from build123d import *

# Parameters (mm, degrees)
SKETCH1_W           = 15.5
SKETCH1_H           = 15.5
BOSS_EXTRUDE1_DEPTH = 6.4
FILLET1_R           = 2.54
FILLET2_R           = 2.54
FILLET3_R           = 2.54
FILLET4_R           = 2.54
SKETCH2_W           = 11
SKETCH2_H           = 11
BOSS_EXTRUDE2_DEPTH = 4
SKETCH3_R           = 5.1
BOSS_EXTRUDE3_DEPTH = 22.9
SKETCH4_W           = 0.7
SKETCH4_H           = 2.8
BOSS_EXTRUDE4_DEPTH = 5.8
CUT_EXTRUDE1_DEPTH  = 35.312716302


with BuildPart() as part:
    # Sketch1 → Boss-Extrude1 (new body)
    with BuildSketch(Plane(origin=(0, 0, 0), x_dir=(1, 0, 0), z_dir=(0, 1, 0))):
        with Locations((7.75, 7.75)):
            Rectangle(SKETCH1_W, SKETCH1_H)
    extrude(amount=BOSS_EXTRUDE1_DEPTH)

    # Fillet1
    fillet1_edges = [part.edges().sort_by_distance(p)[0] for p in [
        (15.5, 3.2, 0),
    ]]
    fillet(fillet1_edges, radius=FILLET1_R)

    # Fillet2
    fillet2_edges = [part.edges().sort_by_distance(p)[0] for p in [
        (0, 3.2, 0),
    ]]
    fillet(fillet2_edges, radius=FILLET2_R)

    # Fillet3
    fillet3_edges = [part.edges().sort_by_distance(p)[0] for p in [
        (15.5, 3.2, -15.5),
    ]]
    fillet(fillet3_edges, radius=FILLET3_R)

    # Fillet4
    fillet4_edges = [part.edges().sort_by_distance(p)[0] for p in [
        (0, 3.2, -15.5),
    ]]
    fillet(fillet4_edges, radius=FILLET4_R)

    # Sketch2 → Boss-Extrude2 (add)
    with BuildSketch(Plane(origin=(0, 6.4, 0), x_dir=(1, 0, 0), z_dir=(0, 1, 0))):
        with Locations((7.75, 7.75)):
            Rectangle(SKETCH2_W, SKETCH2_H)
    extrude(amount=BOSS_EXTRUDE2_DEPTH)

    # Sketch3 → Boss-Extrude3 (add)
    with BuildSketch(Plane.XZ):
        with Locations(Location((7.75, -7.75, 0), (0, 0, 270))):
            Circle(SKETCH3_R)
    extrude(amount=BOSS_EXTRUDE3_DEPTH)

    # Sketch4 → Boss-Extrude4 (add)
    with BuildSketch(Plane.XZ.offset(22.9)):
        with Locations((5.2, -7.75)):
            Rectangle(SKETCH4_W, SKETCH4_H)
        with Locations((10.3, -7.75)):
            Rectangle(SKETCH4_W, SKETCH4_H)
    extrude(amount=BOSS_EXTRUDE4_DEPTH)

    # Sketch5 → Cut-Extrude1 (cut, through all)
    with BuildSketch(Plane(origin=(10.65, 0, 0), x_dir=(0, 0, -1), z_dir=(1, 0, 0))):
        with BuildLine():
            Line((8.489235797, -25.962974619), (8.489235797, -26.848488265))
            ThreePointArc((8.489235797, -26.848488265), (7.75, -27.587724063), (7.010764203, -26.848488265))
            Line((7.010764203, -26.848488265), (7.010764203, -25.962974619))
            ThreePointArc((7.010764203, -25.962974619), (7.75, -25.223738822), (8.489235797, -25.962974619))
        make_face()
    extrude(amount=-CUT_EXTRUDE1_DEPTH, mode=Mode.SUBTRACT)


solid = part.part
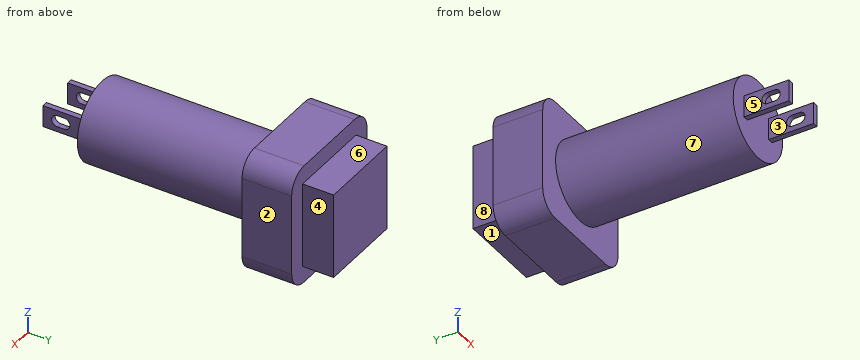
Verification items for the finished model (mm, model axes). Face numbers are marked on the shaded views. A direction names the side the tool comes from. Coordinates: 2 decimals unless noted, no trailing zeros. Order: outer loops, then holes, each group sorted by start corner. A loop starts at its lowest first (then second) coordinate and runs counter-clockwise, first axis right, second up. Notation, with made-up numbers: M 54.5,-17 L 88.5,-17 A26 cw 88.5,22 Z; hole C -36.5,12.25 d11. An arc over 180 degrees is marked long. Write each question's results on one line, items separated by ' | '.
1) Section check C-C on z = -11. Record the cut outline in (x, y), plus the area to 3 significant figures.
Solved:
outline: M 0,0 L 3.82,0 L 3.82,-22.9 L 11.68,-22.9 L 11.68,0 L 15.5,0 L 15.5,6.4 L 13.25,6.4 L 13.25,10.4 L 2.25,10.4 L 2.25,6.4 L 0,6.4 Z | area: 323 mm²
2) Scan lines: line 1 along Y through (x, z) = (5, -11); line 2 along X through (y, z) = (7, -8.75); line 3 along Y through (x, z) = (12.25, -11.5). Record each from-to range of solid material in increasing order. Write a range as [from, to].
Solved:
line 1: y = [-22.9, 10.4] | line 2: x = [2.25, 13.25] | line 3: y = [0, 10.4]
3) Access from +Z, -Z, +X, -X, +Y, -Y to the whole of each face (thin tool, end or side, straight path). Record for the marked faces 4, 5, 6, 7 and 8.
Solved:
face 4: +Z, -Z, +X, +Y | face 5: +Z, -Z, -X, -Y | face 6: +Z, +X, -X, +Y | face 7: -Y | face 8: +Z, -Z, -X, +Y
4) Gauge pin test, flat ends, axial feed: pin 1 Ø6 at (x, y) = (11, -10.5) entering from -Z; pin 2 Ø0.8 at (x, y) = (10.5, -26.5) entering from +Z; pin 3 Ø1.2 at (x, y) = (6.5, 8.5) entering from -Z. Record the tip position at first contact, or that the pin passes through.
Solved:
pin 1: stops at z = -12.84 | pin 2: stops at z = -6.35 | pin 3: stops at z = -13.25
5) Release check for a two-part mould opening along X. For the marked faces 1, 2 and 3 record: pulls with the +X half, pulls with the -X half, needs draft (parallel to the pull), parting line crosses it, or undercut.
Solved:
face 1: needs draft | face 2: pulls with the +X half | face 3: undercut
6) Section check D-D on y = -17. Record the cut outline in (x, z), plus the area to 3 significant figures.
Solved:
outline: C 7.75,-7.75 d10.2 | area: 81.7 mm²
7) Section check A-A on z = -7.75. Record the cut outline in (x, y), plus the area to 3 significant figures.
Solved:
outline: M 0,0 L 2.65,0 L 2.65,-22.9 L 4.85,-22.9 L 4.85,-25.22 L 5.55,-25.22 L 5.55,-22.9 L 9.95,-22.9 L 9.95,-25.22 L 10.65,-25.22 L 10.65,-22.9 L 12.85,-22.9 L 12.85,0 L 15.5,0 L 15.5,6.4 L 13.25,6.4 L 13.25,10.4 L 2.25,10.4 L 2.25,6.4 L 0,6.4 Z; M 4.85,-28.7 L 5.55,-28.7 L 5.55,-27.59 L 4.85,-27.59 Z; M 9.95,-28.7 L 10.65,-28.7 L 10.65,-27.59 L 9.95,-27.59 Z | area: 382 mm²
8) Section check B-B on x = 7.75. Record the cut outline in (y, z), plus the area to 3 significant figures.
Solved:
outline: M -22.9,-12.85 L 0,-12.85 L 0,-15.5 L 6.4,-15.5 L 6.4,-13.25 L 10.4,-13.25 L 10.4,-2.25 L 6.4,-2.25 L 6.4,0 L 0,0 L 0,-2.65 L -22.9,-2.65 Z | area: 377 mm²
